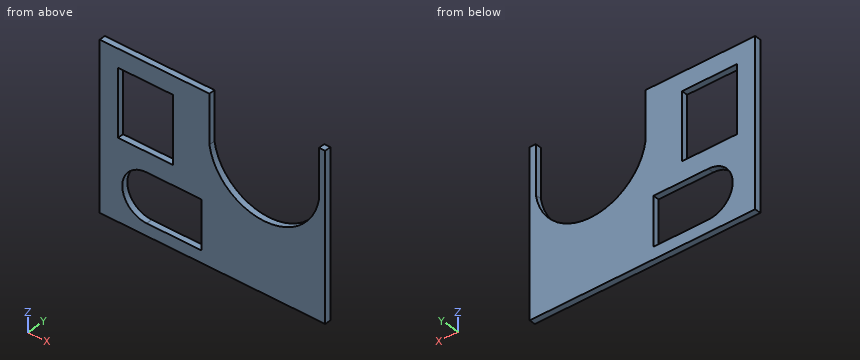
from build123d import *

# Parameters (mm, degrees)
F0_W     = 14.2875
F0_H     = 17.4625
F1_DEPTH = 1.5875


with BuildPart() as f1:
    # F0 (on Front) → F1 (new body)
    with BuildSketch(Plane.XZ):
        with BuildLine():
            Line((-30.1625, 25.4), (-30.1625, -17.78))
            Line((-30.1625, -17.78), (28.575, -17.78))
            Line((28.575, -17.78), (28.575, 25.4))
            Line((28.575, 25.4), (26.9875, 25.4))
            Line((26.9875, 25.4), (26.9875, 12.7))
            ThreePointArc((26.9875, 12.7), (12.7, 0.371714), (-1.5875, 12.7))
            Line((-1.5875, 12.7), (-1.5875, 25.4))
            Line((-1.5875, 25.4), (-30.1625, 25.4))
        make_face()
        with BuildLine():
            ThreePointArc((-17.939954, -14.622975), (-24.289954, -8.272975), (-17.939954, -1.922975))
            Line((-17.939954, -1.922975), (-3.652454, -1.922975))
            Line((-3.652454, -1.922975), (-3.652454, -14.622975))
            Line((-3.652454, -14.622975), (-17.939954, -14.622975))
        make_face(mode=Mode.SUBTRACT)
        with Locations((-18.25625, 11.90625)):
            Rectangle(F0_W, F0_H, mode=Mode.SUBTRACT)
    extrude(amount=F1_DEPTH)


solid = f1.part
CAD build for the part. Positions are in the model's coordinates, mm. Coordinates: 2 decimals unless noted, no trailing zeros. Loops run counter-clockwise (first coordinate to the right, second up) from the corner with the lowest first, then second, coordinate; pieces in that order, holes last. Notation, with made-up numbers: (67.25, 83.5) - (122.25, 83.5) arc R36 cw to (122.25, 117.5) - close; hole circle Ø2 at (43, 11). An arc over 180 degrees is marked (long way). Write item = value, one per line. Start each with the question number.
Q1. Cut at A-A, the plane z = 18.5. List the corners of the cut face in (x, y) (1 decimal).
Q2. Cut at B-B, the plane x = -10. List the corners of the cut face in (y, z).
Q3. Cut at D-D, the plane y = -0.6. Give the number of separate pieces and of enclosed holes in the cut face, then the cut area to 3 significant figures.
Q4. Cut at C-C, the plane x = -17. List the corners of the cut face in (y, z) (1 decimal), then the cut area to 3 significant figures.
Q5. Drill centre lines: L1, parallel to Z at x = -11.5, y = -0.4 (1 decimal); L2, parallel to Z at x = -8, y = -0.45; L3, parallel to X at y = -1.25, z = 12.5 (1 decimal). Where is each one in solid material? Low to high.
Computed:
q1.outline = (-30.2, -1.6) - (-25.4, -1.6) - (-25.4, 0) - (-30.2, 0) - close; (-11.1, -1.6) - (-1.6, -1.6) - (-1.6, 0) - (-11.1, 0) - close; (27, -1.6) - (28.6, -1.6) - (28.6, 0) - (27, 0) - close
q2.outline = (-1.59, -17.78) - (0, -17.78) - (0, -14.62) - (-1.59, -14.62) - close; (-1.59, -1.92) - (0, -1.92) - (0, 25.4) - (-1.59, 25.4) - close
q3.separate_pieces = 1
q3.enclosed_holes = 2
q3.area = 1,410 mm²
q4.outline = (-1.6, -17.8) - (0, -17.8) - (0, -14.6) - (-1.6, -14.6) - close; (-1.6, -1.9) - (0, -1.9) - (0, 3.2) - (-1.6, 3.2) - close; (-1.6, 20.6) - (0, 20.6) - (0, 25.4) - (-1.6, 25.4) - close
q4.area = 20.7 mm²
q5.L1 = -17.8 to -14.6, -1.9 to 3.2, 20.6 to 25.4
q5.L2 = -17.78 to -14.62, -1.92 to 25.4
q5.L3 = -30.2 to -25.4, -11.1 to -1.6, 27 to 28.6
